Part print with two shaded views. Sizes in mm from the minimum x, y, z corner. A direction names the side the tool comes from. Coordinates: 2 decimals unless noted, no trailing zeros. Order: outer loops, then holes, each group sorted by start corner. A loop starts at its lowest first (then second) coordinate and runs counter-clockwise, first axis right, second up. Notation, with made-up numbers: (56.5, 36.5) - (93.5, 36.5) arc R29 cw to (93.5, 69.5) - close; hole circle Ø10 at (24, 61). An arc over 180 degrees is marked (long way). One line per item, written item: value.
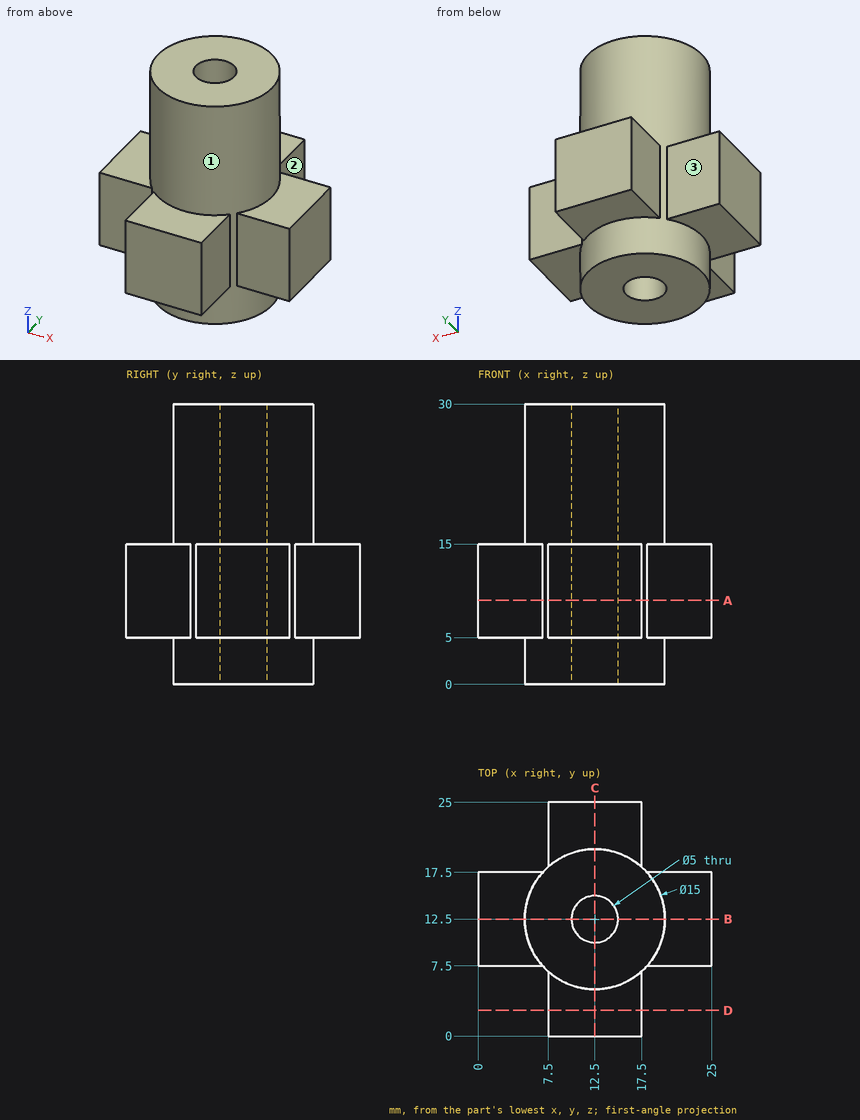
1. Band-saw the part on B-B, the plane y = 12.5. Give the cut face in (x, z), and give its area (3 significant figures).
Values found:
outline: (0, 5) - (5, 5) - (5, 0) - (10, 0) - (10, 30) - (5, 30) - (5, 15) - (0, 15) - close; (15, 0) - (20, 0) - (20, 5) - (25, 5) - (25, 15) - (20, 15) - (20, 30) - (15, 30) - close
area: 400 mm2
2. 3-axis set-ups, long thin cutter, end or side, ignore diameter. For the marked faces 1, 2 and 3: which of +Z, -Z, +X, -X, +Y, -Y reach the whole face in a straight line?
Values found:
face 1: none
face 2: +Z, -Z, +X, +Y
face 3: +Z, -Z, -X, +Y
3. Band-saw the part on D-D, the plane y = 2.75. Give the cut face in (x, z), and give its area (3 significant figures).
Values found:
outline: (7.5, 5) - (17.5, 5) - (17.5, 15) - (7.5, 15) - close
area: 100 mm2
4. Probe line 1 along Y through (x, z) = (1.5, 11.25); line 2 along Z through (x, y) = (2.25, 11). List the from-to ranges inside material, lowest first.
Values found:
line 1: y = 7.5 to 17.5
line 2: z = 5 to 15
5. Band-saw the part on A-A, the plane z = 9. Give the cut face in (x, y).
Values found:
outline: (0, 7.5) - (6.91, 7.5) arc R7.5 ccw to (7.5, 6.91) - (7.5, 0) - (17.5, 0) - (17.5, 6.91) arc R7.5 ccw to (18.09, 7.5) - (25, 7.5) - (25, 17.5) - (18.09, 17.5) arc R7.5 ccw to (17.5, 18.09) - (17.5, 25) - (7.5, 25) - (7.5, 18.09) arc R7.5 ccw to (6.91, 17.5) - (0, 17.5) - close; hole circle Ø5 at (12.5, 12.5)
6. Flat gauge pins, fed straight in: P1, Ø3, axis at x = 4.5, z = 26.5, coming from the -Y side; P2, Ø3.5, axis at y = 4, z = 9.5, coming from the -X side; P3, Ø3.5, axis at x = 5, z = 8, coming from the +Y side. Where does each tip first touch, or does it go through?
Values found:
P1: stops at y = 8.76
P2: stops at x = 7.5
P3: stops at y = 17.5
